Check sheet for the modelled part. Datum: model origin and axes. Units: mm. Face numbers are marked on the shaded views. A direction names the side the tool comes from. Round coordinates to 2 decimals unless told otherwise and drop trailing zeros. Write each loop counter-clockwise with the first axis right and the second up, starting at its lowest first coordinate (ties: lowest second). Pieces come first, ordered by that corner, then holes. Notation, with made-up numbers: (53.5, 37.25) -> (104.5, 37.25) arc R21 cw to (104.5, 61.25) -> close; hole circle Ø3 at (56, 40). An arc over 180 degrees is marked (long way). One line per item, written item: value.
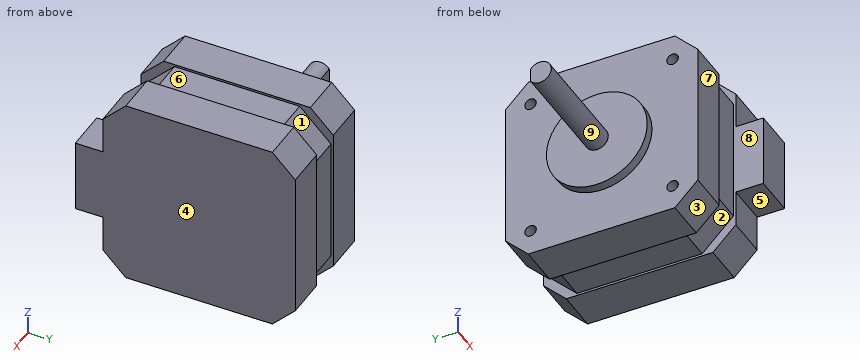
from build123d import *

# Parameters (mm, degrees)
BOSS_EXTRUDE1_DEPTH   = 12.5
CUT_EXTRUDE1_DEPTH    = 3.5
SKETCH4_W             = 7
SKETCH4_H             = 27.34314575
CUT_EXTRUDE2_DEPTH    = 0.5
SKETCH5_W             = 7
SKETCH5_H             = 27.34314575
CUT_EXTRUDE3_DEPTH    = 0.5
SKETCH6_W             = 7
SKETCH6_H             = 27.34314575
CUT_EXTRUDE4_DEPTH    = 0.5
SKETCH7_W             = 7
SKETCH7_H             = 27.34314575
CUT_EXTRUDE5_DEPTH    = 0.5
SKETCH8_R             = 11
BOSS_EXTRUDE2_DEPTH   = 2
SKETCH9_R             = 2.5
BOSS_EXTRUDE3_DEPTH   = 24
M3_TAPPED_HOLE1_D     = 2.5
M3_TAPPED_HOLE1_DEPTH = 6
M3_TAPPED_HOLE1_TIP   = 0.751075774
SKETCH12_W            = 3
SKETCH12_H            = 0.5
CUT_EXTRUDE6_DEPTH    = 20
SKETCH13_W            = 9
SKETCH13_H            = 16
BOSS_EXTRUDE4_DEPTH   = 6


with BuildPart() as part:
    # Sketch1 → Boss-Extrude1 (new body, symmetric)
    with BuildSketch(Plane(origin=(0, 0, 0), x_dir=(0, 0, -1), z_dir=(1, 0, 0))):
        Polygon((-21, 16), (-16, 21), (16, 21), (21, 16), (21, -16), (16, -21), (-16, -21), (-21, -16), align=None)
    extrude(amount=BOSS_EXTRUDE1_DEPTH, both=True)

    # Sketch2 → Cut-Extrude1 (cut, symmetric)
    with BuildSketch(Plane(origin=(0, 0, 0), x_dir=(0, 0, -1), z_dir=(1, 0, 0))):
        Polygon((-21, -13.671572875), (-20.5, -13.671572875), (-13.671572875, -20.5), (-13.671572875, -21), (-16, -21), (-21, -16), align=None)
        Polygon((13.671572875, -21), (13.671572875, -20.5), (20.5, -13.671572875), (21, -13.671572875), (21, -16), (16, -21), align=None)
        Polygon((21, 13.671572875), (20.5, 13.671572875), (13.671572875, 20.5), (13.671572875, 21), (16, 21), (21, 16), align=None)
        Polygon((-13.671572875, 21), (-13.671572875, 20.5), (-20.5, 13.671572875), (-21, 13.671572875), (-21, 16), (-16, 21), align=None)
    extrude(amount=CUT_EXTRUDE1_DEPTH, both=True, mode=Mode.SUBTRACT)

    # Sketch4 → Cut-Extrude2 (cut)
    with BuildSketch(Plane.XY.offset(21)):
        Rectangle(SKETCH4_W, SKETCH4_H)
    extrude(amount=-CUT_EXTRUDE2_DEPTH, mode=Mode.SUBTRACT)

    # Sketch5 → Cut-Extrude3 (cut)
    with BuildSketch(Plane(origin=(0, 21, 0), x_dir=(1, 0, 0), z_dir=(0, 1, 0))):
        Rectangle(SKETCH5_W, SKETCH5_H)
    extrude(amount=-CUT_EXTRUDE3_DEPTH, mode=Mode.SUBTRACT)

    # Sketch6 → Cut-Extrude4 (cut)
    with BuildSketch(Plane(origin=(0, 0, -21), x_dir=(-1, 0, 0), z_dir=(0, 0, -1))):
        Rectangle(SKETCH6_W, SKETCH6_H)
    extrude(amount=-CUT_EXTRUDE4_DEPTH, mode=Mode.SUBTRACT)

    # Sketch7 → Cut-Extrude5 (cut)
    with BuildSketch(Plane.XZ.offset(21)):
        Rectangle(SKETCH7_W, SKETCH7_H)
    extrude(amount=-CUT_EXTRUDE5_DEPTH, mode=Mode.SUBTRACT)

    # Sketch8 → Boss-Extrude2 (add)
    with BuildSketch(Plane.ZY.offset(12.5)):
        Circle(SKETCH8_R)
    extrude(amount=BOSS_EXTRUDE2_DEPTH)

    # Sketch9 → Boss-Extrude3 (add)
    with BuildSketch(Plane.ZY.offset(14.5)):
        Circle(SKETCH9_R)
    extrude(amount=BOSS_EXTRUDE3_DEPTH)

    # M3 Tapped Hole1
    with Locations(Plane.ZY.offset(12.5)):
        with Locations((-15.5, 15.5), (15.5, 15.5), (-15.5, -15.5), (15.5, -15.5)):
            Hole(M3_TAPPED_HOLE1_D / 2, depth=M3_TAPPED_HOLE1_DEPTH)
            with Locations((0, 0, -(M3_TAPPED_HOLE1_DEPTH + M3_TAPPED_HOLE1_TIP / 2))):  # 118° drill point
                Cone(0, M3_TAPPED_HOLE1_D / 2, M3_TAPPED_HOLE1_TIP, mode=Mode.SUBTRACT)

    # Sketch12 → Cut-Extrude6 (cut)
    with BuildSketch(Plane.ZY.offset(38.5)):
        with Locations((0, 2.25)):
            Rectangle(SKETCH12_W, SKETCH12_H)
    extrude(amount=-CUT_EXTRUDE6_DEPTH, mode=Mode.SUBTRACT)

    # Sketch13 → Boss-Extrude4 (add)
    with BuildSketch(Plane.XZ.offset(21)):
        with Locations((8, 0)):
            Rectangle(SKETCH13_W, SKETCH13_H)
    extrude(amount=BOSS_EXTRUDE4_DEPTH)


solid = part.part
Item 1: Mould release check, pull along X, two halves, no side actions. Record for the marked faces 1, 2, 3 and 4: pulls with the +X half, pulls with the -X half, needs draft (parallel to the pull), parting line crosses it, or undercut.
Answer:
face 1: undercut
face 2: undercut
face 3: needs draft
face 4: pulls with the +X half
Item 2: Thickness scan on line 1 (Y direction, x = -10.95, z = 15.5); line 2 (Z direction, x = -3, y = 7.5). Record the ranges inside material, lowest first.
Answer:
line 1: y = -21 to -16.75, -14.25 to 14.25, 16.75 to 21
line 2: z = -20.5 to 20.5
Item 3: Sectioned sample at A-A on y = 0. Enter the section's corners in (x, z).
Answer:
outline: (-38.5, -2.5) -> (-14.5, -2.5) -> (-14.5, -11) -> (-12.5, -11) -> (-12.5, -21) -> (-3.5, -21) -> (-3.5, -20.5) -> (3.5, -20.5) -> (3.5, -21) -> (12.5, -21) -> (12.5, 21) -> (3.5, 21) -> (3.5, 20.5) -> (-3.5, 20.5) -> (-3.5, 21) -> (-12.5, 21) -> (-12.5, 11) -> (-14.5, 11) -> (-14.5, 2.5) -> (-38.5, 2.5) -> close
Item 4: Sectioned sample at C-C on x = -25. Enter the section's corners in (y, z), and give its area (3 significant figures).
Answer:
outline: (2, -1.5) -> (2, 1.5) arc R2.5 ccw (long way) to start
area: 18.6 mm^2
Item 5: Sectioned sample at B-B on z = 0. Enter the section's corners in (x, y).
Answer:
outline: (-38.5, -2.5) -> (-14.5, -2.5) -> (-14.5, -11) -> (-12.5, -11) -> (-12.5, -21) -> (-3.5, -21) -> (-3.5, -20.5) -> (3.5, -20.5) -> (3.5, -27) -> (12.5, -27) -> (12.5, 21) -> (3.5, 21) -> (3.5, 20.5) -> (-3.5, 20.5) -> (-3.5, 21) -> (-12.5, 21) -> (-12.5, 11) -> (-14.5, 11) -> (-14.5, 2.5) -> (-18.5, 2.5) -> (-18.5, 2) -> (-38.5, 2) -> close
Item 6: Tool access check on the marked faces 5, 6, 7, 8 and 9. Record the directions out of +Z, -Z, +X, -X, +Y, -Y that give a thin tool (end or side, any length) a straight path to the whole face; none if there is none.
Answer:
face 5: -Z, +X, -X, -Y
face 6: +Z, +Y, -Y
face 7: +Z, -Z, -X, -Y
face 8: none
face 9: -X
Item 7: Depth check by flat-ended pin: P1, Ø2, axis at x = -9.5, z = -14, coming from the -Y side; P2, Ø4, axis at y = 15.5, z = 15.5, coming from the -X side; P3, Ø1.5, axis at x = -31, z = -0.5, coming from the +Y side. Enter the tip coordinate at first touch or a pass-through.
Answer:
P1: stops at y = -21
P2: stops at x = -12.5
P3: stops at y = 2
Item 8: Sectioned sample at D-D on y = 12. Enter the section's corners in (x, z), and give its area (3 significant figures).
Answer:
outline: (-12.5, -21) -> (-3.5, -21) -> (-3.5, -20.5) -> (3.5, -20.5) -> (3.5, -21) -> (12.5, -21) -> (12.5, 21) -> (3.5, 21) -> (3.5, 20.5) -> (-3.5, 20.5) -> (-3.5, 21) -> (-12.5, 21) -> close
area: 1,040 mm^2
